The listing builds one solid part. Answer for the finished solid, in the listing's coordinates (mm). A direction names the side the tool comes from. Coordinates: 2 decimals unless noted, no trailing zeros. Loops run counter-clockwise (first coordinate to the right, second up) from the corner with the lowest first, then second, coordinate; pieces in that order, holes last. Notation, with made-up numbers: (-10.5, -21) - (37.5, -21) arc R17 ccw to (37.5, 11) - close; hole circle Ø5 at (-35.5, 79). An arc over 180 degrees is marked (long way). Return JSON: item names as keys, results as strings. Group by question number.
1. Section A-A (z = 31) is taken. Write down the section's boundary in (x, y), and give its area (3 significant figures).
2. Which of the six approach directions +Z, -Z, +X, -X, +Y, -Y give full straight-line access (tool end or side, diameter ignored) to faces 1 (the face through (0.813, -42.551, 11.172)), 2 (the face through (36.4, 22, 1.5)), 3 (the face through (-2.75, -12.4, 156.71)), 4 (the face through (0.813, -42.472, 1.449)), 5 (the face through (-37.43, 23.14, 6.33))?
3. Find the intervals of material crossed by line 1 along Z through (x, y) = (-58, -26); line 2 along X through (y, z) = (3, 173.5); line 3 along Y through (x, z) = (6, 226), in increasing order.
```python
from build123d import *

# Parameters (mm, degrees)
F1_DEPTH = 12.7
F2_R     = 12.7
F3_DEPTH = 304.8
F4_R     = 5.08
F5_R     = 5.08


with BuildPart() as f1:
    # F0 (on Top) → F1 (new body)
    with BuildSketch(Plane.XY):
        Polygon((0.525394, 87.986612), (-76.461339, -43.538301), (75.935944, -44.448311), align=None)
    extrude(amount=F1_DEPTH)

    # F2 (on Top) → F3 (join)
    with BuildSketch(Plane.XY):
        Circle(F2_R)
    extrude(amount=F3_DEPTH)

    # F4
    f4_edges = [f1.edges().sort_by_distance(p)[0] for p in [
        (-37.967972, 22.224156, 12.7),
        (38.230669, 21.769151, 12.7),
        (-0.262697, -43.993306, 12.7),
    ]]
    fillet(f4_edges, radius=F4_R)

    # F5
    f5_edges = [f1.edges().sort_by_distance(p)[0] for p in [
        (38.230669, 21.769151, 0),
        (-37.967972, 22.224156, 0),
        (-0.262697, -43.993306, 0),
    ]]
    fillet(f5_edges, radius=F5_R)


solid = f1.part
```
The answers:
{
 "1": {"outline": "circle Ø25.4 at (0, 0)", "area": "507 mm2"},
 "2": {"face 1": "+Z, -X, -Y", "face 2": "-Z, +X, +Y", "face 3": "+Z", "face 4": "-Z, -X, -Y", "face 5": "+Z, -Z, -X, +Y"},
 "3": {"line 1": "z = 0 to 12.7", "line 2": "x = -12.34 to 12.34", "line 3": "y = -11.19 to 11.19"}
}
